```python
from build123d import *

# Parameters (mm, degrees)
F0_R      = 2.54
F0_R_2    = 3.175
F5_DEPTH  = 9
F6_R      = 1.5875
F7_DEPTH  = 2.54
F8_R      = 6.35
F9_DEPTH  = 5.08
F10_R     = 6.35
F11_DEPTH = 5.08


with BuildPart() as f4:
    # F1 (on Front) → F4 section 0
    with BuildSketch(Plane.XZ):
        with BuildLine():
            ThreePointArc((38.1, 17.05), (37.514214, 18.464214), (36.1, 19.05))
            Line((36.1, 19.05), (-36.1, 19.05))
            ThreePointArc((-36.1, 19.05), (-37.514214, 18.464214), (-38.1, 17.05))
            Line((-38.1, 17.05), (-38.1, -17.05))
            ThreePointArc((-38.1, -17.05), (-37.514214, -18.464214), (-36.1, -19.05))
            Line((-36.1, -19.05), (36.1, -19.05))
            ThreePointArc((36.1, -19.05), (37.514214, -18.464214), (38.1, -17.05))
            Line((38.1, -17.05), (38.1, 17.05))
        make_face()
    # F3 (on offset) → F4 section 1
    with BuildSketch(Plane.XZ.offset(-9)):
        with BuildLine():
            Line((36.1, 26.05), (-36.1, 26.05))
            ThreePointArc((-36.1, 26.05), (-42.463961, 23.413961), (-45.1, 17.05))
            Line((-45.1, 17.05), (-45.1, -17.05))
            ThreePointArc((-45.1, -17.05), (-42.463961, -23.413961), (-36.1, -26.05))
            Line((-36.1, -26.05), (36.1, -26.05))
            ThreePointArc((36.1, -26.05), (42.463961, -23.413961), (45.1, -17.05))
            Line((45.1, -17.05), (45.1, 17.05))
            ThreePointArc((45.1, 17.05), (42.463961, 23.413961), (36.1, 26.05))
        make_face()
    loft()

    # F0 (on Front) → F5 (cut, through all)
    with BuildSketch(Plane.XZ):
        with Locations((31.75, -12.7)):
            Circle(F0_R)
        with Locations((31.75, 12.7)):
            Circle(F0_R)
        with Locations((-31.75, -12.7)):
            Circle(F0_R)
        with Locations((-31.75, 12.7)):
            Circle(F0_R)
        Circle(F0_R_2)
    extrude(amount=-F5_DEPTH, mode=Mode.SUBTRACT)

    # F6 (on face) → F7 (cut)
    with BuildSketch(Plane.XZ):
        with Locations((31.75, 0)):
            Circle(F6_R)
        with Locations((-31.75, 0)):
            Circle(F6_R)
    extrude(amount=-F7_DEPTH, mode=Mode.SUBTRACT)

    # F8 (on face) → F9 (cut)
    with BuildSketch(Plane.XZ):
        Circle(F8_R)
    extrude(amount=-F9_DEPTH, mode=Mode.SUBTRACT)

    # F10 (on face) → F11 (cut)
    with BuildSketch(Plane(origin=(0, 9, 0), x_dir=(-1, 0, 0), z_dir=(0, 1, 0))):
        with Locations((-31.75, 12.7)):
            Circle(F10_R)
        with Locations((-31.75, -12.7)):
            Circle(F10_R)
        with Locations((31.75, 12.7)):
            Circle(F10_R)
        with Locations((31.75, -12.7)):
            Circle(F10_R)
    extrude(amount=-F11_DEPTH, mode=Mode.SUBTRACT)


solid = f4.part
```
For this review, take the finished solid that the model builds, in its own axes (mm). A direction names the side the tool comes from. Round coordinates to 2 decimals unless told otherwise and drop trailing zeros. Write each loop counter-clockwise with the first axis right and the second up, starting at its lowest first coordinate (ties: lowest second). Pieces come first, ordered by that corner, then holes.
1) Take a section at D-D on z = 12.7. Give the boundary of the cut face in (x, y), then the cut area to 3 significant figures.
Answer below:
outline: (-45.1, 9) - (-38.1, 0) - (-34.29, 0) - (-34.29, 3.92) - (-38.1, 3.92) - (-38.1, 9) - close; (-29.21, 0) - (29.21, 0) - (29.21, 3.92) - (25.4, 3.92) - (25.4, 9) - (-25.4, 9) - (-25.4, 3.92) - (-29.21, 3.92) - close; (34.29, 0) - (38.1, 0) - (45.1, 9) - (38.1, 9) - (38.1, 3.92) - (34.29, 3.92) - close
area: 580 mm2
2) For line 1 along Z through (x, y) = (31.75, 3); line 2 along Z through (x, y) = (-31.75, 7.25); line 3 along Y through (x, z) = (22, -23), list the stretches that pass through material, from the lowest coordinate up.
Answer below:
line 1: z = -21.38 to -15.24, -10.16 to 10.16, 15.24 to 21.38
line 2: z = -24.69 to -19.05, -6.35 to 6.35, 19.05 to 24.69
line 3: y = 5.08 to 9
3) Take a section at A-A on x = 0. Give the boundary of the cut face in (y, z) (3 decimals).
Answer below:
outline: (0, -19.05) - (9, -26.05) - (9, -3.175) - (5.08, -3.175) - (5.08, -6.35) - (0, -6.35) - close; (0, 6.35) - (5.08, 6.35) - (5.08, 3.175) - (9, 3.175) - (9, 26.05) - (0, 19.05) - close
4) Machinability: for faces 1 (the face through (41.649, 4.563, -0.239)), 2 (the face through (31.8, 3.92, -15.4)), 3 (the face through (33.264, 1.252, 0.477)), which of the approach directions +Z, -Z, +X, -X, +Y, -Y give a long, thin tool a straight path to every point of the face, cutting with its end or side? Answer none if there is none.
Answer below:
face 1: +Z, -Z, +X, -Y
face 2: +Y
face 3: -Y
5) Take a section at C-C on x = -31.75. Give the boundary of the cut face in (y, z), then the cut area to 3 significant figures.
Answer below:
outline: (0, -19.05) - (9, -26.05) - (9, -19.05) - (3.92, -19.05) - (3.92, -15.24) - (0, -15.24) - close; (0, -10.16) - (3.92, -10.16) - (3.92, -6.35) - (9, -6.35) - (9, 6.35) - (3.92, 6.35) - (3.92, 10.16) - (0, 10.16) - (0, 1.59) - (2.54, 1.59) - (2.54, -1.59) - (0, -1.59) - close; (0, 15.24) - (3.92, 15.24) - (3.92, 19.05) - (9, 19.05) - (9, 26.05) - (0, 19.05) - close
area: 229 mm2
6) Insertion check: pin 1 Ø1.5 at (y, z) = (4.5, 16) entering from -X; pin 2 Ø14 at (x, z) = (-32.5, -11.5) entering from +Y; pin 3 Ø1 at (x, z) = (32.5, -0.5) entering from -Y; pin 4 Ø6.5 at (x, z) = (-31.75, -12.7) entering from +Y. Each pin has a flat end and moves straight along its axis. Give the tip position at first contact, or say it passes through.
Answer below:
pin 1: stops at x = -42.18
pin 2: stops at y = 9
pin 3: stops at y = 2.54
pin 4: stops at y = 3.92
7) Mouldability with a two-part tool opening along Z and no side actions: class faces 4 (the face through (-41.649, 4.563, 0.239)), 5 (the face through (-0.505, 4.563, -22.599)), 6 (the face through (32, 2.54, 0)) as +Z half, -Z half, draft (parallel to the pull), parting line (faces both ways), or undercut.
Answer below:
face 4: draft
face 5: -Z half
face 6: undercut
